Check sheet for the modelled part. Datum: model origin and axes. Units: mm. A direction names the side the tool comes from. Round coordinates to 2 decimals unless told otherwise and drop trailing zeros. Write each loop counter-clockwise with the first axis right and the second up, starting at its lowest first coordinate (ties: lowest second). Pieces come first, ordered by that corner, then holes. Notation, with made-up numbers: M 23,18.25 L 32,18.25 A6 cw 32,28.25 Z; hole C -19.5,-12 d3. An arc over 180 degrees is marked long. Answer in a Markdown table with one row per item.
Autodesk Inventor part; units mm, degrees
ref_plane "Start plane" through (0, 0, 60) normal (0, 0, 1) x (1, 0, 0)
ref_plane "End plane" through (0, 0, 1940) normal (0, 0, 1) x (1, 0, 0)
ref_plane "Work Plane4" through (-50, -150, 1940) normal (0, 0, 1) x (1, 0, 0)
ref_plane "Start plane" through (0, 0, 60) normal (0, 0, 1) x (1, 0, 0)
ref_plane "End plane" through (0, 0, 1940) normal (0, 0, 1) x (1, 0, 0)
sketch "Sketch" plane through (0, 0, 0) normal (0, 0, 1) x (1, 0, 0)
  line L0 (-50, -40) -> (-50, 40)
  line L1 (-40, 50) -> (40, 50)
  line L2 (50, 40) -> (50, -40)
  line L3 (40, -50) -> (-40, -50)
  arc A0 (-50, -40) -> (-40, -50) centre (-40, -40) ccw
  arc A1 (50, 40) -> (40, 50) centre (40, 40) ccw
  arc A2 (-40, 50) -> (-50, 40) centre (-40, 40) ccw
  arc A3 (40, -50) -> (50, -40) centre (40, -40) ccw
  arc A4 (-40, 45) -> (-45, 40) centre (-40, 40) ccw
  line L4 (-40, 45) -> (40, 45)
  arc A5 (45, 40) -> (40, 45) centre (40, 40) ccw
  line L5 (45, 40) -> (45, -40)
  arc A6 (40, -45) -> (45, -40) centre (40, -40) ccw
  line L6 (40, -45) -> (-40, -45)
  arc A7 (-45, -40) -> (-40, -45) centre (-40, -40) ccw
  line L7 (-45, -40) -> (-45, 40)
  line L8 (0, 72.8995) -> (0, -72.8995) construction
  line L9 (-72.8995, 0) -> (72.8995, 0) construction
  dimension "d7" = 10
  dimension "d9" = 100
  dimension "d11" = 100
  dimension "d12" = 5
  dimension "d15" = 50
  dimension "d16" = 50
extrude "Body" add sketch "Sketch" along normal up to surface (1880 mm away) from surface at 60
sketch "Sketch3" plane through (0, 0, 0) normal (0, 0, 1) x (1, 0, 0)
  line L0 (0, 0) -> (10, 0)
ref_plane "Work Plane3" through (0, 0, 0) normal (0, -1, 0) x (1, 0, 0)
ref_plane "Work Plane4" through (-50, -150, 1940) normal (0, 0, 1) x (1, 0, 0)
split "Split1" plane through (-50, -150, 1940) removes the side toward (0, 0, 1)
ref_plane "Work Plane5" through (50, -150, 60) normal (0, 0, -1) x (-1, 0, 0)
split "Split2" plane through (50, -150, 60) removes the side toward (0, 0, -1)
sketch "Sketch4" plane through (0, 0, 0) normal (0, -1, 0) x (1, 0, 0)
  line L0 (-2, 60) -> (12, 60)
  line L1 (-2, 1940) -> (12, 1940)
  dimension "d18" = 1880
equation "\"d7\" = G_IR"
equation "\"d9\" = G_W"
equation "\"d11\" = G_H"
equation "\"d12\" = G_T"
equation "\"d15\" = 0.5 * d9"
equation "\"d16\" = 0.5 * d11"
equation "\"d3\" = G_L"
equation "\"G_W\" = 100"
equation "\"G_H\" = 100"
equation "\"G_T\" = 5"
equation "\"G_IR\" = 10"
equation "\"G_L\" = d18"
properties part number "ISO 10799-2 - 100x100x5 - 1880" material "Steel, Mild"
1. Section check A-A, the plane x = 4. Record the cut outline in (y, z), and give its area (3 significant figures).
Found:
| item | result |
|---|---|
| outline | M -50,60 L -45,60 L -45,1940 L -50,1940 Z; M 45,60 L 50,60 L 50,1940 L 45,1940 Z |
| area | 18,800 mm2 |
2. Access from +Z, -Z, +X, -X, +Y, -Y to the whole of each face (thin tool, end or side, straight path). Record for faces 5 (the face through (-1, 50, 987)), 6 (the face through (1, -45, 987)).
Found:
| item | result |
|---|---|
| face 5 | +Z, -Z, +X, -X, +Y |
| face 6 | +Z, -Z |
3. Section check C-C, the plane z = 592. Record the cut outline in (x, y).
Found:
| item | result |
|---|---|
| outline | M -50,-40 A10 ccw -40,-50 L 40,-50 A10 ccw 50,-40 L 50,40 A10 ccw 40,50 L -40,50 A10 ccw -50,40 Z; hole M -45,-40 A5 ccw -40,-45 L 40,-45 A5 ccw 45,-40 L 45,40 A5 ccw 40,45 L -40,45 A5 ccw -45,40 Z |
4. Draft check along X on faces 1 (the face through (45, 1, 987)), 2 (the face through (-4, -48, 1940)), 3 (the face through (-50, -1, 987)), 4 (the face through (-45, -1, 987)). Enter one of: +X half, -X half, draft (parallel to the pull), parting line (faces both ways), or undercut.
Found:
| item | result |
|---|---|
| face 1 | undercut |
| face 2 | draft |
| face 3 | -X half |
| face 4 | undercut |
5. Scan lines: L1, parallel to Y at x = 21, z = 619; L2, parallel to X at y = -41.5, z = 1451.5. Record each from-to range of solid material in increasing order.
Found:
| item | result |
|---|---|
| L1 | y = -50 to -45, 45 to 50 |
| L2 | x = -49.89 to -44.77, 44.77 to 49.89 |
